Autodesk Inventor part; units mm, degrees
ref_plane "YZ Plane" through (0, 0, 0) normal (1, 0, 0) x (0, 1, 0)
ref_plane "XZ Plane" through (0, 0, 0) normal (0, 1, 0) x (-1, 0, 0)
ref_plane "XY Plane" through (0, 0, 0) normal (0, 0, 1) x (1, 0, 0)
sketch "Sketch1" plane through (0, 0, 0) normal (0, 1, 0) x (-1, 0, 0)
  line L0 (0, 0) -> (56, 0)
  line L1 (56, 0) -> (56, 60)
  line L2 (56, 60) -> (0, 60)
  line L3 (0, 60) -> (0, 0)
  circle A0 centre (7.25, 5) radius 1.25
  circle A1 centre (7.25, 45) radius 1.25
  line L4 (28, 60) -> (28, 0) construction
  circle A2 centre (48.75, 5) radius 1.25
  circle A3 centre (48.75, 45) radius 1.25
  dimension "d0" = 56
  dimension "d1" = 60
  dimension "d4" = 2.5
  dimension "d5" = 7.25
  dimension "d6" = 5
  dimension "d7" = 2.5
  dimension "d8" = 7.25
  dimension "d9" = 40
extrude "Extrusion1" add sketch "Sketch1" along normal blind 3
properties part number "wall-front-outer-scaled"
Model file for the job. Use its own axes, mm. Coordinates: 2 decimals unless noted, no trailing zeros. Write each loop counter-clockwise with the first axis right and the second up, starting at its lowest first coordinate (ties: lowest second). Pieces come first, ordered by that corner, then holes. Notation, with made-up numbers: (61, -31.75) - (111, -31.75) arc R20 cw to (111, 2.25) - close; hole circle Ø1 at (19.5, 42). An arc over 180 degrees is marked (long way). One line per item, written item: value. Start each with the question number.
1. Slice it at B-B (x = -48.75). Write the cut outline in (y, z).
2. Probe line 1 (Z direction, x = -48.75, y = 2.1); line 2 (Z direction, x = -49.5, y = 2.4). List the from-to ranges inside material, lowest first. Write a range as from..to.
3. Slice it at A-A (z = 45). Write the cut outline in (x, y), plus the area to 3 significant figures.
4. Flat gauge pin, fed straight in: pin 1 (2 mm diameter, centred on x = -48.75, z = 5, fed in from +Y). Where does the tip first touch, or does it go through?
5. Mould opens along Z. For faces 1 (the flat face through (-28, 3, 30)), 2 (the cylindrical face through (-7.09, 1.48, 43.76)), 3 (the flat face through (-28, 1, 0)) say: released by +Z, released by -Z, zero draft, split by the parting line, or undercut.
Answers below:
1. outline: (0, 0) - (3, 0) - (3, 3.75) - (0, 3.75) - close; (0, 6.25) - (3, 6.25) - (3, 43.75) - (0, 43.75) - close; (0, 46.25) - (3, 46.25) - (3, 60) - (0, 60) - close
2. line 1: z = 0..3.75, 6.25..43.75, 46.25..60
2. line 2: z = 0..4, 6..44, 46..60
3. outline: (-56, 0) - (-50, 0) - (-50, 3) - (-56, 3) - close; (-47.5, 0) - (-8.5, 0) - (-8.5, 3) - (-47.5, 3) - close; (-6, 0) - (0, 0) - (0, 3) - (-6, 3) - close
3. area: 153 mm^2
4. pin 1: passes through
5. face 1: zero draft
5. face 2: undercut
5. face 3: released by -Z
